Geometry: see drawing. Coordinates: mm, zero at the bounding-box minimum. A direction names the side the tool comes from. Give positions to 0.01 mm unless a question says otherwise; leave off trailing zeros. Loops run counter-clockwise (first coordinate to the right, second up) from the corner with the lowest first, then second, coordinate; pieces in that order, holes last. Notation, with made-up numbers: M 83.25,68 L 108.25,68 A27 cw 108.25,91 Z; hole C 31,88.5 d2. An arc over 180 degrees is marked long. Use CSV: the item, a comma, the result in double quotes. Start each with the question number.
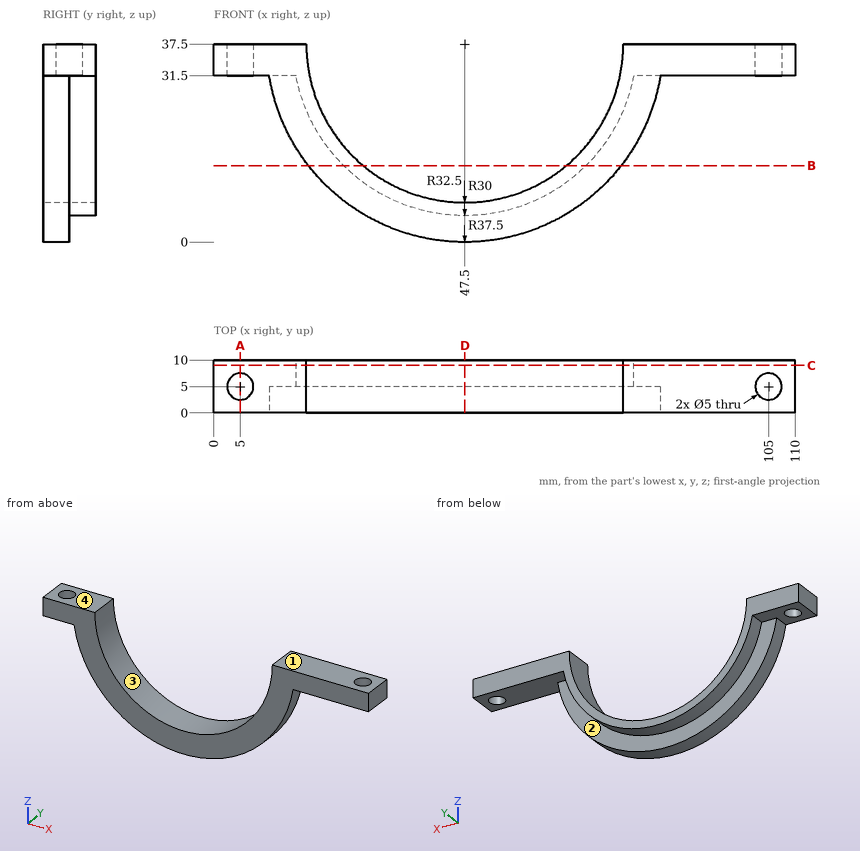
Item 1: Mould query, pull axis X, two halves, no side actions, for the marked faces 3 and 4. Classes: +X half, -X half, draft (parallel to the pull), parting line (faces both ways), or undercut.
Item 2: Section D-D (x = 47.5). Output: boundary loops of the cut face in (y, z).
Item 3: Section A-A (x = 5). Output: boundary loops of the cut face in (y, z), then the cut area to 3 significant figures.
Item 4: Material intervals for line 1 (Y direction, x = 5, z = 36); line 2 (X direction, y = 4.5, z = 33); line 3 (Z direction, x = 98.5, y = 3.5), sorted ascending.
Item 5: Section C-C (y = 9). Output: boundary loops of the cut face in (x, z), then the cut area to 3 significant figures.
Item 6: Section B-B (z = 14.5). Output: boundary loops of the cut face in (x, y).
Item 7: Set-up query: the marked faces 1 and 2. Return all of +Z, -Z, +X, -X, +Y, -Y with unobstructed straight access to the full face (end or side cutting, diameter ignored); none if empty.
Item 8: First-contact query: pin 1 Ø3 at (x, y) = (95.5, 6) entering from -Z; pin 2 Ø3 at (y, z) = (7, 26) entering from -X; pin 3 Ø5 at (y, z) = (5, 9.5) entering from -X; pin 4 Ø6 at (x, y) = (105, 5) entering from +Z. Flat tips, straight axial feed; report the tip coordinate or a pass-through.
Recorded:
1,face 3,"undercut"
1,face 4,"draft"
2,outline,"M 0,0 L 5,0 L 5,5 L 10,5 L 10,7.5 L 0,7.5 Z"
3,outline,"M 0,31.5 L 2.5,31.5 L 2.5,37.5 L 0,37.5 Z; M 7.5,31.5 L 10,31.5 L 10,37.5 L 7.5,37.5 Z"
3,area,"30.0 mm²"
4,line 1,"0 to 2.5, 7.5 to 10"
4,line 2,"0 to 2.55, 7.45 to 17.84, 77.16 to 102.55, 107.45 to 110"
4,line 3,"31.5 to 37.5"
5,outline,"M 0,31.5 L 15.56,31.5 A32.5 ccw 79.44,31.5 L 110,31.5 L 110,37.5 L 77.5,37.5 A30 cw 17.5,37.5 L 0,37.5 Z"
5,area,"518 mm²"
6,outline,"M 17.88,0 L 28.24,0 L 28.24,10 L 24.54,10 L 24.54,5 L 17.88,5 Z; M 66.76,0 L 77.12,0 L 77.12,5 L 70.46,5 L 70.46,10 L 66.76,10 Z"
7,face 1,"+Z, +X, -X, +Y, -Y"
7,face 2,"-Z, +Y"
8,pin 1,"z = 31.5"
8,pin 2,"x = 16.58"
8,pin 3,"x = 20"
8,pin 4,"z = 37.5"
